Model file for the job. Use its own axes, mm. A direction names the side the tool comes from. Give positions to 0.01 mm unless a question says otherwise; leave off trailing zeros. Order: outer loops, then holes, each group sorted by start corner. A loop starts at its lowest first (then second) coordinate and runs counter-clockwise, first axis right, second up. Notation, with made-up numbers: M -16.75,-22.5 L 13.25,-22.5 A35 cw 13.25,16.5 Z; hole C 22,74.25 d8. An arc over 180 degrees is marked long. Return JSON: item names as keys, results as strings. Group by question number.
1. 3-axis set-ups, long thin cutter, end or side, ignore diameter. For faces 1 (the face through (0, -2, 0)), 2 (the face through (0, 0.95, -1)), 3 (the face through (-1.1, 1, 13.9)): which of +Z, -Z, +X, -X, +Y, -Y reach the whole face in a straight line?
2. Slice it at A-A on x = 0. List the corners of the cut face in (y, z).
3. Slice it at C-C on y = -1.25. List the corners of the cut face in (x, z).
4. Two-plate mould, pull along Y, no slides. Class faces 4 (the face through (0, 0, 21)), 5 (the face through (0, -0.95, -1)), 6 (the face through (0.62, 3.85, 0.99)): released by +Y, released by -Y, zero draft, split by the parting line, or undercut.
5. Wall check: probe 1 along Y at (x, z) = (0, 0.8); probe 2 along Z at (x, y) = (0.1, 2.75); probe 3 along Z at (x, y) = (-1.2, -1). Give the ranges that are in metal, low to high. Write a range as [from, to].
6. Pin check, flat tips, straight feed: pin 1 (3 mm diameter, centred on x = -0.5, y = 3.5, fed in from +Z); pin 2 (3 mm diameter, centred on y = 1.5, z = 12, fed in from -X); pin 3 (2 mm diameter, centred on x = 1.5, z = 11, fed in from -Y). Stop position of each tip, or through.
7. Slice it at D-D on z = 10.5. List the corners of the cut face in (x, y) (1 decimal).
8. Slice it at B-B on z = 4. List the corners of the cut face in (x, y).
from build123d import *

# Parameters (mm, degrees)
SKETCH1_R           = 1.35
BOSS_EXTRUDE1_DEPTH = 2
SKETCH2_R           = 2.5
BOSS_EXTRUDE2_DEPTH = 5
SKETCH3_R           = 1.4875
BOSS_EXTRUDE3_DEPTH = 14
BOSS_EXTRUDE4_START = 2
BOSS_EXTRUDE4_DEPTH = 2
CHAMFER1_SIZE       = 0.5


with BuildPart() as part:
    # Sketch1 → Boss-Extrude1 (new body)
    with BuildSketch(Plane.XY):
        with BuildLine():
            Line((-2.5, 5.05), (-2.5, 0))
            ThreePointArc((-2.5, 0), (0, -2.5), (2.5, 0))
            Line((2.5, 0), (2.5, 5.05))
            ThreePointArc((2.5, 5.05), (0, 7.55), (-2.5, 5.05))
        make_face()
        with Locations((0, 5.05)):
            Circle(SKETCH1_R, mode=Mode.SUBTRACT)
    extrude(amount=BOSS_EXTRUDE1_DEPTH)

    # Sketch2 → Boss-Extrude2 (add)
    with BuildSketch(Plane.XY.offset(2)):
        Circle(SKETCH2_R)
    extrude(amount=BOSS_EXTRUDE2_DEPTH)

    # Sketch3 → Boss-Extrude3 (add)
    with BuildSketch(Plane.XY.offset(7)):
        Circle(SKETCH3_R)
    extrude(amount=BOSS_EXTRUDE3_DEPTH)

    # Sketch4 → Boss-Extrude4 (add)
    with BuildSketch(Plane(origin=(0, 0, 0), x_dir=(-1, 0, 0), z_dir=(0, 0, -1)).offset(BOSS_EXTRUDE4_START)):
        with BuildLine():
            Line((-2.5, 0), (-2.5, 0.95))
            Line((-2.5, 0.95), (2.5, 0.95))
            Line((2.5, 0.95), (2.5, 0))
            ThreePointArc((2.5, 0), (2.4526685, -0.484166531), (2.312466216, -0.95))
            Line((2.312466216, -0.95), (-2.312466216, -0.95))
            ThreePointArc((-2.312466216, -0.95), (-2.4526685, -0.484166531), (-2.5, 0))
        make_face()
    extrude(amount=-BOSS_EXTRUDE4_DEPTH)

    # Chamfer1
    chamfer1_edges = [part.edges().sort_by_distance(p)[0] for p in [
        (0, -0.95, -2),
        (0, 0.95, -2),
    ]]
    chamfer(chamfer1_edges, length=CHAMFER1_SIZE)


solid = part.part
Result:
{
 "1": {"face 1": "-Z, +X, -X, -Y", "face 2": "-Z, +X, -X, +Y", "face 3": "+Z"},
 "2": {"outline": "M -2.5,0 L -0.95,0 L -0.95,-1.5 L -0.45,-2 L 0.45,-2 L 0.95,-1.5 L 0.95,0 L 3.7,0 L 3.7,2 L 2.5,2 L 2.5,7 L 1.49,7 L 1.49,21 L -1.49,21 L -1.49,7 L -2.5,7 Z; M 6.4,0 L 7.55,0 L 7.55,2 L 6.4,2 Z"},
 "3": {"outline": "M -2.17,0 L 2.17,0 L 2.17,7 L 0.81,7 L 0.81,21 L -0.81,21 L -0.81,7 L -2.17,7 Z"},
 "4": {"face 4": "zero draft", "face 5": "released by -Y", "face 6": "undercut"},
 "5": {"probe 1": "y = [-2.5, 3.7], [6.4, 7.55]", "probe 2": "z = [0, 2]", "probe 3": "z = [0, 7]"},
 "6": {"pin 1": "stops at z = 7", "pin 2": "stops at x = -1.49", "pin 3": "stops at y = -1.4"},
 "7": {"outline": "C 0,0 d3"},
 "8": {"outline": "C 0,0 d5"}
}
